Geometry: see drawing. Coordinates: mm, zero at the bounding-box minimum. A direction names the side the tool comes from. Give positions to 0.01 mm unless a question says otherwise; leave off trailing zeros. Loops run counter-clockwise (first coordinate to the right, second up) from the corner with the lowest first, then second, coordinate; pieces in that order, holes last. Notation, with made-up numbers: (53, 34.5) -> (84, 34.5) arc R25 cw to (84, 56.5) -> close; hole circle Ø10 at (-27.5, 80.25). An arc over 180 degrees is marked (long way). Return JSON: item names as keys, results as strings. Group by question number.
(1) Pin query (flat end, axial travel): pin 1 (3 mm diameter, centred on x = 30, z = 9.5, fed in from -Y); pin 2 (1 mm diameter, centred on y = 9.5, z = 7.5, fed in from -X); pin 3 (3.5 mm diameter, centred on x = 1.5, z = 7, fed in from +Y); pin 4 (1.5 mm diameter, centred on x = 2, z = 2.5, fed in from -Y). Return the tip coordinate at first contact, or that it passes through.
(2) Cut plane D-D on x = 10.35. Return loops of the section in (y, z).
(3) Cut plane A-A on x = 2. Return loops of the section in (y, z), then the cut area to 3 significant figures.
(4) Cut plane B-B on z = 2.5. Return loops of the section in (x, y).
(5) Cut plane C-C on z = 6. Return loops of the section in (x, y).
(6) Access query for the marked faces 1, 2 and 3. Directions: +Z, -Z, +X, -X, +Y, -Y. A direction counts if a zero-diameter tool reaches every point of the face in a straight line with its end or side. Return the directions, or none.
(7) Ray query, line 1 (X direction, y = 20.4, z = 2.5); line 2 (X direction, y = 14.5, z = 6); line 3 (Y direction, x = 25.5, z = 3.75). Return the intervals inside material, ascending. Write a range as from..to.
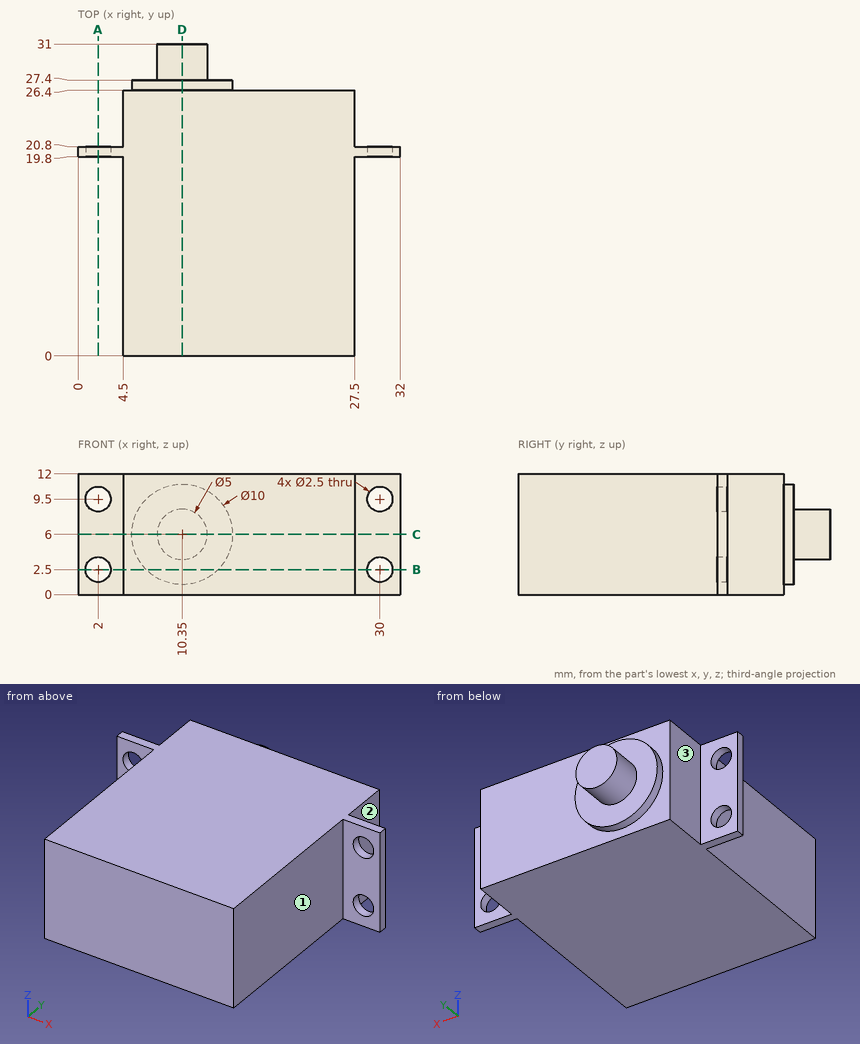
Answers:
{
 "1": {"pin 1": "y = 19.8", "pin 2": "x = 4.5", "pin 3": "y = 20.8", "pin 4": "through"},
 "2": {"outline": "(0, 0) -> (26.4, 0) -> (26.4, 1) -> (27.4, 1) -> (27.4, 3.5) -> (31, 3.5) -> (31, 8.5) -> (27.4, 8.5) -> (27.4, 11) -> (26.4, 11) -> (26.4, 12) -> (0, 12) -> close"},
 "3": {"outline": "(19.8, 0) -> (20.8, 0) -> (20.8, 1.25) -> (19.8, 1.25) -> close; (19.8, 3.75) -> (20.8, 3.75) -> (20.8, 8.25) -> (19.8, 8.25) -> close; (19.8, 10.75) -> (20.8, 10.75) -> (20.8, 12) -> (19.8, 12) -> close", "area": "7.00 mm²"},
 "4": {"outline": "(0, 19.8) -> (0.75, 19.8) -> (0.75, 20.8) -> (0, 20.8) -> close; (3.25, 19.8) -> (4.5, 19.8) -> (4.5, 0) -> (27.5, 0) -> (27.5, 19.8) -> (28.75, 19.8) -> (28.75, 20.8) -> (27.5, 20.8) -> (27.5, 26.4) -> (13.92, 26.4) -> (13.92, 27.4) -> (6.78, 27.4) -> (6.78, 26.4) -> (4.5, 26.4) -> (4.5, 20.8) -> (3.25, 20.8) -> close; (31.25, 19.8) -> (32, 19.8) -> (32, 20.8) -> (31.25, 20.8) -> close"},
 "5": {"outline": "(0, 19.8) -> (4.5, 19.8) -> (4.5, 0) -> (27.5, 0) -> (27.5, 19.8) -> (32, 19.8) -> (32, 20.8) -> (27.5, 20.8) -> (27.5, 26.4) -> (15.35, 26.4) -> (15.35, 27.4) -> (12.85, 27.4) -> (12.85, 31) -> (7.85, 31) -> (7.85, 27.4) -> (5.35, 27.4) -> (5.35, 26.4) -> (4.5, 26.4) -> (4.5, 20.8) -> (0, 20.8) -> close"},
 "6": {"face 1": "+Z, -Z, +X, -Y", "face 2": "+Z, -Z, +X, +Y", "face 3": "+Z, -Z, -X, +Y"},
 "7": {"line 1": "0..0.75, 3.25..28.75, 31.25..32", "line 2": "4.5..27.5", "line 3": "0..26.4"}
}
